Could you check a few things on this model? Use its own coordinates, in mm. Face numbers are marked on the shaded views. Give positions to 0.01 mm unless a question says otherwise; leave off trailing zeros. Order: outer loops, then holes, each group sorted by start corner. A loop starts at its lowest first (then second) coordinate and runs counter-clockwise, first axis right, second up. Notation, with made-up numbers: M 28.25,-23.5 L 63.25,-23.5 A17 cw 63.25,-14.5 Z; hole C 62,39 d10. An arc over 180 degrees is marked long. Use a Markdown table: item, result. Add a question column.
Item 1: Suppose I cut it at C-C on z = 3.35. Write out the boundary of the cut face in (x, y).
Item 2: Suppose I cut it at A-A on x = 0. Write out the boundary of the cut face in (y, z), plus the area to 3 significant figures.
Item 3: Suppose I cut it at B-B on y = 0. Write out the boundary of the cut face in (x, z), plus the area to 3 significant figures.
Item 4: If we mould it in two halves opening along Y, with no side actions, what happens to the marked faces 1, 2 and 3? For each: released by +Y, released by -Y, zero draft, split by the parting line, or undercut.
Item 5: Suppose I cut it at D-D on x = -20.5. Write out the boundary of the cut face in (y, z).
Item 6: If I drill on L1, parallel to Y at x = 1, z = 3.3; L2, parallel to X at y = 6, z = 2.3; L3, parallel to Y at x = -3.5, z = 0.9, over which ranges is the centre line in solid material (lowest first)? Write a range as from..to.
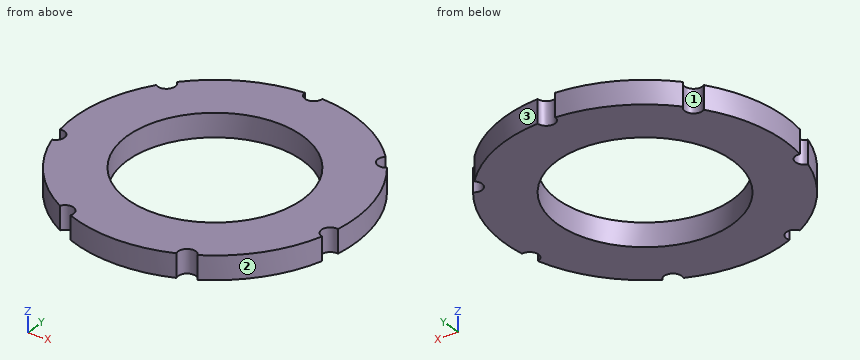
from build123d import *

# Parameters (mm, degrees)
SKETCH1_R           = 15
BOSS_EXTRUDE1_DEPTH = 4


with BuildPart() as part:
    # Sketch1 → Boss-Extrude1 (new body)
    with BuildSketch(Plane.XY):
        with BuildLine():
            ThreePointArc((-1.499267399, 23.953125), (-10.413209739, 21.62325283), (-17.792529295, 16.106703613))
            ThreePointArc((-17.792529295, 16.106703613), (-17.591208356, 14.028520542), (-19.662085162, 13.762354707))
            ThreePointArc((-19.662085162, 13.762354707), (-23.398269892, 5.340502415), (-23.686188528, -3.868394111))
            ThreePointArc((-23.686188528, -3.868394111), (-21.935878024, -5.006721014), (-23.018951765, -6.791749381))
            ThreePointArc((-23.018951765, -6.791749381), (-18.763955579, -14.963755245), (-11.74366469, -20.930512169))
            ThreePointArc((-11.74366469, -20.930512169), (-9.76238413, -20.271799528), (-9.042078187, -22.231527659))
            ThreePointArc((-9.042078187, -22.231527659), (0, -24), (9.042078187, -22.231527659))
            ThreePointArc((9.042078187, -22.231527659), (9.76238413, -20.271799528), (11.74366469, -20.930512169))
            ThreePointArc((11.74366469, -20.930512169), (18.763955579, -14.963755245), (23.018951765, -6.791749381))
            ThreePointArc((23.018951765, -6.791749381), (21.935878024, -5.006721014), (23.686188528, -3.868394111))
            ThreePointArc((23.686188528, -3.868394111), (23.398269892, 5.340502415), (19.662085162, 13.762354707))
            ThreePointArc((19.662085162, 13.762354707), (17.591208356, 14.028520542), (17.792529295, 16.106703613))
            ThreePointArc((17.792529295, 16.106703613), (10.413209739, 21.62325283), (1.499267399, 23.953125))
            ThreePointArc((1.499267399, 23.953125), (0, 22.5), (-1.499267399, 23.953125))
        make_face()
        Circle(SKETCH1_R, mode=Mode.SUBTRACT)
    extrude(amount=BOSS_EXTRUDE1_DEPTH)


solid = part.part
Findings below:
| question | item | result |
|---|---|---|
| 1 | outline | M -23.69,-3.87 A1.5 cw -23.02,-6.79 A24 ccw -11.74,-20.93 A1.5 cw -9.04,-22.23 A24 ccw 9.04,-22.23 A1.5 cw 11.74,-20.93 A24 ccw 23.02,-6.79 A1.5 cw 23.69,-3.87 A24 ccw 19.66,13.76 A1.5 cw 17.79,16.11 A24 ccw 1.5,23.95 A1.5 cw -1.5,23.95 A24 ccw -17.79,16.11 A1.5 cw -19.66,13.76 A24 ccw Z; hole C 0,0 d30 |
| 2 | outline | M -24,0 L -15,0 L -15,4 L -24,4 Z; M 15,0 L 22.5,0 L 22.5,4 L 15,4 Z |
| 2 | area | 66.0 mm^2 |
| 3 | outline | M -24,0 L -15,0 L -15,4 L -24,4 Z; M 15,0 L 24,0 L 24,4 L 15,4 Z |
| 3 | area | 72.0 mm^2 |
| 4 | face 1 | undercut |
| 4 | face 2 | released by -Y |
| 4 | face 3 | released by +Y |
| 5 | outline | M -12.48,0 L 12.48,0 L 12.48,4 L -12.48,4 Z |
| 6 | L1 | y = -23.98..-14.97, 14.97..22.88 |
| 6 | L2 | x = -23.24..-13.75, 13.75..23.24 |
| 6 | L3 | y = -23.74..-14.59, 14.59..23.74 |
